Geometry: see drawing. Coordinates: mm, zero at the bounding-box minimum. Round coordinates to 2 decimals unless told otherwise and drop trailing zeros. Loops run counter-clockwise (first coordinate to the right, second up) from the corner with the lowest first, then second, coordinate; pieces in that order, holes last. Notation, with made-up numbers: (31.5, 48.5) - (79.5, 48.5) arc R29 cw to (79.5, 83.5) - close; hole circle Ø4 at (63.25, 80.5). An arc over 180 degrees is marked (long way). Return JSON: item names as keys, results as strings. Group by question number.
1. Section C-C on x = 26.5. Return loops of the section in (y, z), and give its area (3 significant figures).
2. Material intervals for probe 1 along Y at (x, z) = (86, 4.25); probe 2 along X at (y, z) = (201.5, 3.8); probe 3 along X at (y, z) = (15, 5.2), sorted ascending.
3. Section D-D on y = 40.5. Return loops of the section in (x, z), and give its area (3 significant figures).
4. Section A-A on x = 65. Return loops of the section in (y, z), and give its area (3 significant figures).
5. First-contact query: pin 1 Ø1.8 at (x, z) = (76, 3) entering from -Y; pin 2 Ø1.2 at (y, z) = (13, 3) entering from -X; pin 3 Ø1.2 at (y, z) = (209, 4) entering from -X. Flat tips, straight axial feed; report the tip coordinate or a pass-through.
6. Section B-B on z = 3.8. Return loops of the section in (x, y), and give its area (3 significant figures).
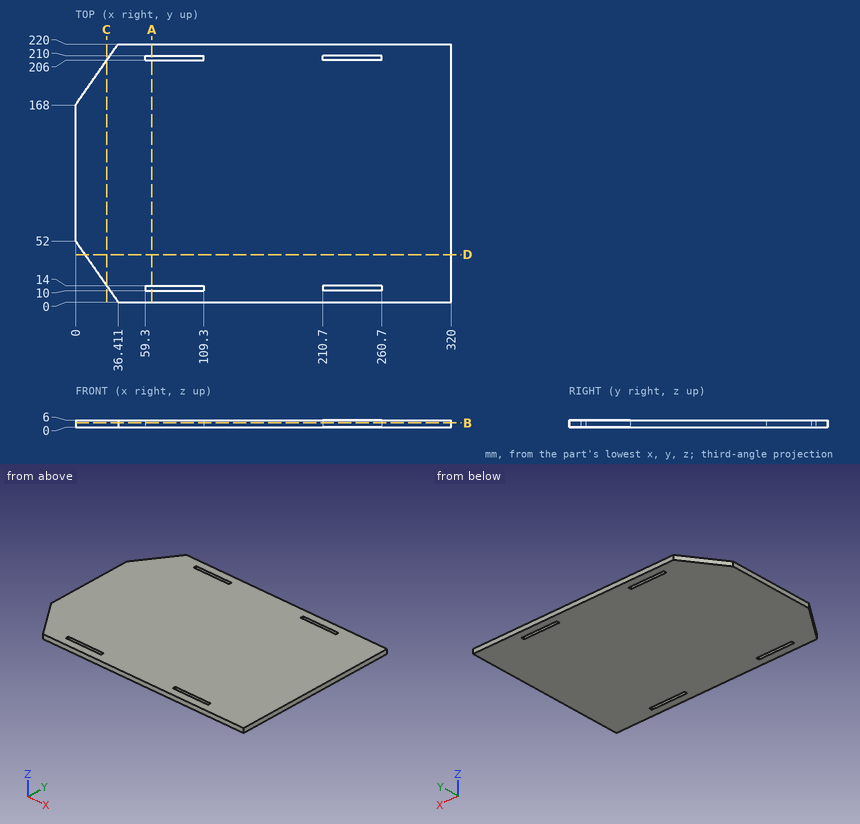
Taken from the geometry:
{
 "1": {"outline": "(14.15, 0) - (205.85, 0) - (205.85, 6) - (14.15, 6) - close", "area": "1,150 mm2"},
 "2": {"probe 1": "0 to 10, 14 to 206, 210 to 220", "probe 2": "23.46 to 320", "probe 3": "25.91 to 320"},
 "3": {"outline": "(8.05, 0) - (320, 0) - (320, 6) - (8.05, 6) - close", "area": "1,870 mm2"},
 "4": {"outline": "(0, 0) - (10, 0) - (10, 6) - (0, 6) - close; (14, 0) - (206, 0) - (206, 6) - (14, 6) - close; (210, 0) - (220, 0) - (220, 6) - (210, 6) - close", "area": "1,270 mm2"},
 "5": {"pin 1": "y = 0", "pin 2": "x = 26.89", "pin 3": "x = 28.29"},
 "6": {"outline": "(0, 52) - (36.41, 0) - (320, 0) - (320, 220) - (36.41, 220) - (0, 168) - close; hole (59.3, 10) - (109.3, 10) - (109.3, 14) - (59.3, 14) - close; hole (59.3, 206) - (109.3, 206) - (109.3, 210) - (59.3, 210) - close; hole (210.7, 10) - (260.7, 10) - (260.7, 14) - (210.7, 14) - close; hole (210.7, 206) - (260.7, 206) - (260.7, 210) - (210.7, 210) - close", "area": "67,700 mm2"}
}
